Geometry: final body of the model. Coordinates: model frame, mm. Face numbers are marked on the shaded views. A direction names the side the tool comes from. Round coordinates to 2 decimals unless told otherwise and drop trailing zeros. Loops run counter-clockwise (first coordinate to the right, second up) from the corner with the lowest first, then second, coordinate; pieces in that order, holes last. Notation, with made-up numbers: M 11.25,-1.75 L 23.25,-1.75 A29 cw 23.25,19.25 Z; hole C 38.5,77.5 d10. An arc over 180 degrees is marked long. Answer as a JSON object with one key per item and string values.
Autodesk Inventor part; units mm, degrees
ref_plane "YZ Plane" through (0, 0, 0) normal (1, 0, 0) x (0, 1, 0)
ref_plane "XZ Plane" through (0, 0, 0) normal (0, 1, 0) x (-1, 0, 0)
ref_plane "XY Plane" through (0, 0, 0) normal (0, 0, 1) x (1, 0, 0)
sketch "Sketch5" plane through (0, 0, 0) normal (1, 0, 0) x (0, 1, 0)
  line L0 (0, 0) -> (0, 14)
  line L1 (0, 14) -> (3, 14)
  line L2 (3, 14) -> (3, 4)
  line L3 (3, 4) -> (8.8859, 4)
  line L4 (8.8859, 4) -> (21.9322, 11.8789)
  line L5 (21.9322, 11.8789) -> (24, 8.4549)
  line L6 (24, 8.4549) -> (10, 0)
  line L7 (10, 0) -> (0, 0)
  dimension "d31" = 3
  dimension "d32" = 4
  dimension "d33" = 4
  dimension "d34" = 14
  dimension "d35" = 10
  dimension "d36" = 10
extrude "Extrusion4" add sketch "Sketch5" along normal blind 30
sketch "Sketch6" plane through (0, 3, 14) normal (0, 1, 0) x (1, 0, 0)
  circle A0 centre (5, 5) radius 1.5
  circle A1 centre (25, 5) radius 1.5
  line L0 (30, 10) -> (30, 0)
  line L1 (0, 0) -> (30, 0)
  line L2 (0, 0) -> (0, 10)
  point P0 (0, 14)
  dimension "d39" = 3
  dimension "d40" = 3
  dimension "d41" = 5
  dimension "d42" = 5
  dimension "d43" = 5
  dimension "d44" = 5
extrude "Extrusion5" cut sketch "Sketch6" against normal blind 30
fillet "Fillet5" radius 5 2 edges at (0, 1.5, 14) (30, 1.5, 14)
sketch "Sketch7" plane through (30, 24, 8.4549) normal (0, 0.517, -0.856) x (-1, 0, 0)
  arc A0 (8.5, -9) -> (5.5, -9) centre (7, -7) ccw
  arc A1 (24.5, -9) -> (21.5, -9) centre (23, -7) ccw
  line L0 (30, 0) -> (30, -16.355)
  line L1 (30, 0) -> (0, 0)
  line L2 (0, -16.355) -> (0, 0)
  line L3 (5.5, -9) -> (8.5, -9)
  line L4 (21.5, -9) -> (24.5, -9)
  point P0 (30, -24.9151)
  dimension "d48" = 5
  dimension "d49" = 5
  dimension "d50" = 7
  dimension "d51" = 7
  dimension "d52" = 7
  dimension "d53" = 7
  dimension "d54" = 4.5
extrude "Extrusion6" cut sketch "Sketch7" against normal blind 30
fillet "Fillet6" radius 7 2 edges at (0, 22.9661, 10.1669) (30, 22.9661, 10.1669)
sketch "Sketch8" plane through (0, 8.8859, 4) normal (0, -0.517, 0.856) x (1, 0, 0)
  arc A0 (8.5, 6.2408) -> (5.5, 6.2408) centre (7, 8.2408) ccw
  circle A1 centre (7, 8.2408) radius 3.25
  arc A2 (24.5, 6.2408) -> (21.5, 6.2408) centre (23, 8.2408) ccw
  circle A3 centre (23, 8.2408) radius 3.25
  point P0 (0, -9.6742)
  dimension "d58" = 6.5
  dimension "d59" = 6.5
extrude "Extrusion7" cut sketch "Sketch8" against normal blind 0.8
fillet "Fillet7" radius 2 1 edges at (15, 3, 4)
fillet "Fillet8" radius 12 2 edges at (15, 8.8859, 4) (15, 10, 0)
fillet "Fillet9" radius 1.5 9 edges at (15, 24, 8.4549) (2.0503, 22.245, 7.395) (0, 15.4345, 3.282) (0, 9.8774, 0.44) (0, 3.3288, 0) (30, 15.4345, 3.282) (30, 9.8774, 0.44) (30, 3.3288, 0) (27.9497, 22.245, 7.395)
fillet "Fillet10" radius 1.5 14 edges at (30, 13.8435, 6.9941) (27.9497, 20.1771, 10.819) (15, 21.9322, 11.8789) (2.0503, 20.1771, 10.819) (0, 13.8435, 6.9941) (0, 8.7633, 4.44) (0, 5.2717, 4) (0, 3, 7.5) (1.4645, 3, 12.5355) (15, 3, 14) (28.5355, 3, 12.5355) (30, 3, 7.5) (30, 5.2717, 4) (30, 8.7633, 4.44)
fillet "Fillet11" radius 0.5 8 edges at (29.5607, 0, 0.4393) (15, 0, 0) (0.4393, 0, 0.4393) (0, 0, 5.25) (1.4645, 0, 12.5355) (15, 0, 14) (28.5355, 0, 12.5355) (30, 0, 5.25)
properties part number "SwitchMount"
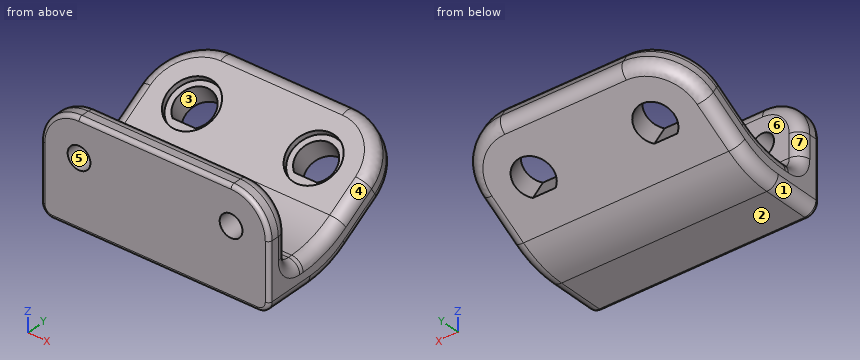
1) Section query A-A (x = 17.5). Return the cut outline in (y, z).
Results:
{"outline": "M 0,0.5 A0.5 ccw 0.5,0 L 6.66,0 A12 ccw 12.86,1.73 L 22.72,7.68 A1.5 ccw 23.22,9.74 L 22.71,10.59 A1.5 ccw 20.65,11.1 L 11.75,5.73 A12 cw 5.54,4 L 5,4 A2 cw 3,6 L 3,12.5 A1.5 ccw 1.5,14 L 0.5,14 A0.5 ccw 0,13.5 Z"}
2) Ray query, line 1 (X direction, y = 0.75, z = 9); line 2 (Z direction, x = 5, y = 0.95); line 3 (Y direction, x = 28, z = 7.75). Return the intervals inside material, ascending.
Results:
{"line 1": "0 to 3.5, 6.5 to 23.5, 26.5 to 30", "line 2": "0 to 7.5, 10.5 to 14", "line 3": "0 to 3, 15.1 to 21.54"}
3) Pin query (flat end, axial travel): P1, Ø10, axis at x = 27, y = 7.5, coming from the +Z side; P2, Ø3, axis at x = 3.5, y = 21, coming from the -Z side; P3, Ø1, axis at x = 13, y = 8.5, coming from the +Z side. Return the tip coordinate at first contact, or that it passes through.
Results:
{"P1": "z = 13.41", "P2": "z = 5.74", "P3": "z = 4.51"}
4) Reachability of the marked faces 4, 5, 6 and 7 from +Z, -Z, +X, -X, +Y, -Y: full face, straight path, thin tool, end or side. Return the list, or none.
Results:
{"face 4": "+Z, +X", "face 5": "-Y", "face 6": "+Z, +X, -X", "face 7": "+Z, -X"}
5) Pull-direction query (X, two-part tool) for the marked faces 1, 2 and 3; classes: +X half, -X half, draft (parallel to the pull), parting line (faces both ways), or undercut.
Results:
{"face 1": "-X half", "face 2": "draft", "face 3": "undercut"}
